from build123d import *

# Parameters (mm, degrees)
SKETCH1_W                     = 165.1
SKETCH1_H                     = 38.1
BOSS_EXTRUDE1_DEPTH           = 82.55
BOSS_EXTRUDE2_START           = 19.05
SKETCH1_3_R                   = 15
BOSS_EXTRUDE2_DEPTH           = 28.575
BOSS_EXTRUDE3_START           = -47.625
SKETCH1_5_R                   = 15
BOSS_EXTRUDE3_DEPTH           = 28.575
SKETCH2_R                     = 26
CUT_EXTRUDE1_DEPTH            = 36.83
SKETCH2_3_R                   = 76.2
SKETCH2_3_R_2                 = 69.85
CUT_EXTRUDE2_DEPTH            = 8
M14X2_0_TAPPED_HOLE1_REACH    = 224.273
M14X2_0_TAPPED_HOLE1_BORE_R   = 6
F_1_0MM_DOWEL_HOLE1_OUTLINE_R = 6.35
F_1_0MM_DOWEL_HOLE1_DEPTH     = 20.05
F_1_0MM_DOWEL_HOLE2_D         = 12.7
FILLET1_R                     = 3.175
FILLET2_R                     = 3.175


# Read off the part's stored shape, not the designer's step: Ø1.0mm Dowel Hole1
with BuildPart() as part:
    # Sketch1 → Boss-Extrude1 (new, symmetric)
    with BuildSketch(Plane.XY):
        with Locations((0, 19.05)):
            Rectangle(SKETCH1_W, SKETCH1_H)
    extrude(amount=BOSS_EXTRUDE1_DEPTH, both=True)

    # Sketch1<3> → Boss-Extrude2 (add)
    with BuildSketch(Plane.XY.offset(BOSS_EXTRUDE2_START)):
        with BuildLine():
            Line((-47.625, 76.2), (-47.625, 38.1))
            Line((-47.625, 38.1), (47.625, 38.1))
            Line((47.625, 38.1), (47.625, 76.2))
            ThreePointArc((47.625, 76.2), (0, 123.825), (-47.625, 76.2))
        make_face()
        with Locations((0, 76.2)):
            Circle(SKETCH1_3_R, mode=Mode.SUBTRACT)
    extrude(amount=BOSS_EXTRUDE2_DEPTH)

    # Sketch1<5> → Boss-Extrude3 (add)
    with BuildSketch(Plane.XY.offset(BOSS_EXTRUDE3_START)):
        with BuildLine():
            Line((-47.625, 76.2), (-47.625, 38.1))
            Line((-47.625, 38.1), (47.625, 38.1))
            Line((47.625, 38.1), (47.625, 76.2))
            ThreePointArc((47.625, 76.2), (0, 123.825), (-47.625, 76.2))
        make_face()
        with Locations((0, 76.2)):
            Circle(SKETCH1_5_R, mode=Mode.SUBTRACT)
    extrude(amount=BOSS_EXTRUDE3_DEPTH)

    # Sketch2 → Cut-Extrude1 (cut)
    with BuildSketch(Plane.XZ):
        Circle(SKETCH2_R)
    extrude(amount=-CUT_EXTRUDE1_DEPTH, mode=Mode.SUBTRACT)

    # Sketch2<3> → Cut-Extrude2 (cut)
    with BuildSketch(Plane.XZ):
        Circle(SKETCH2_3_R)
        Circle(SKETCH2_3_R_2, mode=Mode.SUBTRACT)
    extrude(amount=-CUT_EXTRUDE2_DEPTH, mode=Mode.SUBTRACT)

    # M14x2.0 Tapped Hole1 bore → M14x2.0 Tapped Hole1 (cut, up to next)
    with BuildSketch(Plane.ZY.offset(82.55), mode=Mode.PRIVATE) as m14x2_0_tapped_hole1_sk1:
        with Locations((0, 20.05)):
            Circle(M14X2_0_TAPPED_HOLE1_BORE_R)
    m14x2_0_tapped_hole1_tool1 = extrude(m14x2_0_tapped_hole1_sk1.sketch, amount=-M14X2_0_TAPPED_HOLE1_REACH, mode=Mode.PRIVATE) & part.part
    add(m14x2_0_tapped_hole1_tool1.solids().sort_by_distance((-82.55, 20.05, 0))[0], mode=Mode.SUBTRACT)

    # Ø1.0mm Dowel Hole1 outline → Ø1.0mm Dowel Hole1 (cut)
    with BuildSketch(Plane(origin=(0, 0, 0), x_dir=(1, 0, 0), z_dir=(0, 1, 0))):
        with Locations((-50.55, 0)):
            Circle(F_1_0MM_DOWEL_HOLE1_OUTLINE_R)
    extrude(amount=F_1_0MM_DOWEL_HOLE1_DEPTH, mode=Mode.SUBTRACT)

    # Ø1.0mm Dowel Hole2 (through all)
    with Locations(Plane(origin=(0, 38.1, 0), x_dir=(1, 0, 0), z_dir=(0, 1, 0))):
        with Locations((-61.963767235, 61.963767235), (61.963767235, -61.963767235), (-61.963767235, -61.963767235), (61.963767235, 61.963767235)):
            Hole(F_1_0MM_DOWEL_HOLE2_D / 2)

    # Fillet1
    fillet1_edges = [part.edges().sort_by_distance(p)[0] for p in [
        (82.55, 19.05, 82.55),
        (-82.55, 19.05, 82.55),
        (82.55, 19.05, -82.55),
        (-82.55, 19.05, -82.55),
    ]]
    fillet(fillet1_edges, radius=FILLET1_R)

    # Fillet2
    fillet2_edges = [part.edges().sort_by_distance(p)[0] for p in [
        (0, 38.1, -82.55),
        (82.55, 38.1, 0),
        (-82.55, 38.1, 0),
        (0, 38.1, 82.55),
        (-81.62006403, 38.1, 81.62006403),
        (81.62006403, 38.1, 81.62006403),
        (-81.62006403, 38.1, -81.62006403),
        (81.62006403, 38.1, -81.62006403),
        (0, 123.825, 47.625),
        (-47.625, 57.15, 47.625),
        (0, 38.1, 19.05),
        (-47.625, 38.1, 33.3375),
        (47.625, 57.15, 47.625),
        (47.625, 38.1, 33.3375),
        (0, 38.1, 47.625),
        (0, 123.825, 19.05),
        (47.625, 57.15, 19.05),
        (-47.625, 57.15, 19.05),
        (0, 123.825, -19.05),
        (47.625, 57.15, -19.05),
        (0, 38.1, -47.625),
        (47.625, 38.1, -33.3375),
        (-47.625, 57.15, -19.05),
        (-47.625, 38.1, -33.3375),
        (0, 123.825, -47.625),
        (47.625, 57.15, -47.625),
        (-47.625, 57.15, -47.625),
        (0, 38.1, -19.05),
    ]]
    fillet(fillet2_edges, radius=FILLET2_R)


solid = part.part
Build history of the part. All positions in model axes, mm. A direction names the side the tool comes from. Round coordinates to 2 decimals unless told otherwise and drop trailing zeros. Loops run counter-clockwise (first coordinate to the right, second up) from the corner with the lowest first, then second, coordinate; pieces in that order, holes last. Notation, with made-up numbers: (59, 5.25) -> (67, 5.25) arc R26 ccw to (67, 26.25) -> close; hole circle Ø2 at (24.25, 27.25). An arc over 180 degrees is marked (long way). One line per item, written item: value. Start each with the question number.
Q1. Probe line 1 along Z through (x, y) = (29, 62) (3 decimals); line 2 along Y through (x, z) = (0, -30.25) (3 decimals); line 3 along Y through (x, z) = (-42, 0). List the from-to ranges inside material, lowest first.
Q2. Drop flat-ended pins along their axis: pin 1 Ø6.5 at (y, z) = (52.5, 31.5) entering from +X (3 decimals); pin 2 Ø12 at (x, y) = (65, 41.5) entering from -Z; pin 3 Ø1.5 at (x, z) = (54.5, 42.5) entering from -Y; pin 4 Ø24 at (x, y) = (21.5, 84.5) entering from +Z (3 decimals). Give the stop position or say it passes through.
Q3. Cut at B-B on z = 0. List the corners of the cut face in (x, y) (3 decimals).
Q4. Cut at C-C on x = 0. Count the separate pieces of the cut face and the enclosed holes in it, plus the area to 3 significant figures.
Q5. 3-axis set-ups, long thin cutter, end or side, ignore diameter. For faces 5 (the face through (34, 8, -62)), 6 (the face through (-47.625, 59, -33)), 7 (the face through (9, 90, 19.05)), 8 (the face through (-54.32, 26, -0.78)): which of +Z, -Z, +X, -X, +Y, -Y reach the whole face in a straight line?
Q6. Two-plate mould, pull along X, no slides. Class faces 1 (the face through (82.55, 17, 1)), 2 (the face through (9, 90, 47.625)), 3 (the face through (59.03, 18.78, -56.33)), 4 (the face through (-1.953, 91.072, -33.538)): released by +X, released by -X, zero draft, split by the parting line, or undercut.
Q7. Cut at D-D on z = -32. List the corners of the cut face in (x, y) (3 decimals), plus the area to 3 significant figures.
Q8. Cut at A-A on y = 44.5. List the corners of the cut face in (x, z) (3 decimals), plus the area to 3 significant figures.
Computed:
1. line 1: -47.625 to -19.05, 19.05 to 47.625
1. line 2: 0 to 61.2, 91.2 to 123.825
1. line 3: 0 to 14.05, 26.05 to 38.1
2. pin 1: x = 47.625
2. pin 2: z = -82.5
2. pin 3: y = 0
2. pin 4: z = 47.625
3. outline: (-82.55, 0) -> (-76.2, 0) -> (-76.2, 8) -> (-69.85, 8) -> (-69.85, 0) -> (-56.9, 0) -> (-56.9, 14.05) -> (-82.55, 14.05) -> close; (-82.55, 26.05) -> (-26, 26.05) -> (-26, 36.83) -> (26, 36.83) -> (26, 0) -> (69.85, 0) -> (69.85, 8) -> (76.2, 8) -> (76.2, 0) -> (82.55, 0) -> (82.55, 34.925) arc R3.175 ccw to (79.375, 38.1) -> (-79.375, 38.1) arc R3.175 ccw to (-82.55, 34.925) -> close; (-44.2, 0) -> (-26, 0) -> (-26, 14.05) -> (-44.2, 14.05) -> close
4. separate pieces: 3
4. enclosed holes: 0
4. area: 7,450 mm²
5. face 5: -Y
5. face 6: +Z, -Z, -X, +Y
5. face 7: +X, -X, +Y
5. face 8: -X
6. face 1: released by +X
6. face 2: zero draft
6. face 3: undercut
6. face 4: undercut
7. outline: (-82.55, 0) -> (-69.155, 0) -> (-69.155, 8) -> (-62.089, 8) -> (-62.089, 0) -> (62.089, 0) -> (62.089, 8) -> (69.155, 8) -> (69.155, 0) -> (82.55, 0) -> (82.55, 34.925) arc R3.175 ccw to (79.375, 38.1) -> (50.8, 38.1) arc R3.175 cw to (47.625, 41.275) -> (47.625, 76.2) arc R47.625 ccw to (-47.625, 76.2) -> (-47.625, 41.275) arc R3.175 cw to (-50.8, 38.1) -> (-79.375, 38.1) arc R3.175 ccw to (-82.55, 34.925) -> close; hole circle Ø30 at (0, 76.2)
7. area: 12,700 mm²
8. outline: (-47.625, -44.45) arc R3.175 ccw to (-44.45, -47.625) -> (44.45, -47.625) arc R3.175 ccw to (47.625, -44.45) -> (47.625, -22.225) arc R3.175 ccw to (44.45, -19.05) -> (-44.45, -19.05) arc R3.175 ccw to (-47.625, -22.225) -> close; (-47.625, 22.225) arc R3.175 ccw to (-44.45, 19.05) -> (44.45, 19.05) arc R3.175 ccw to (47.625, 22.225) -> (47.625, 44.45) arc R3.175 ccw to (44.45, 47.625) -> (-44.45, 47.625) arc R3.175 ccw to (-47.625, 44.45) -> close
8. area: 5,430 mm²
